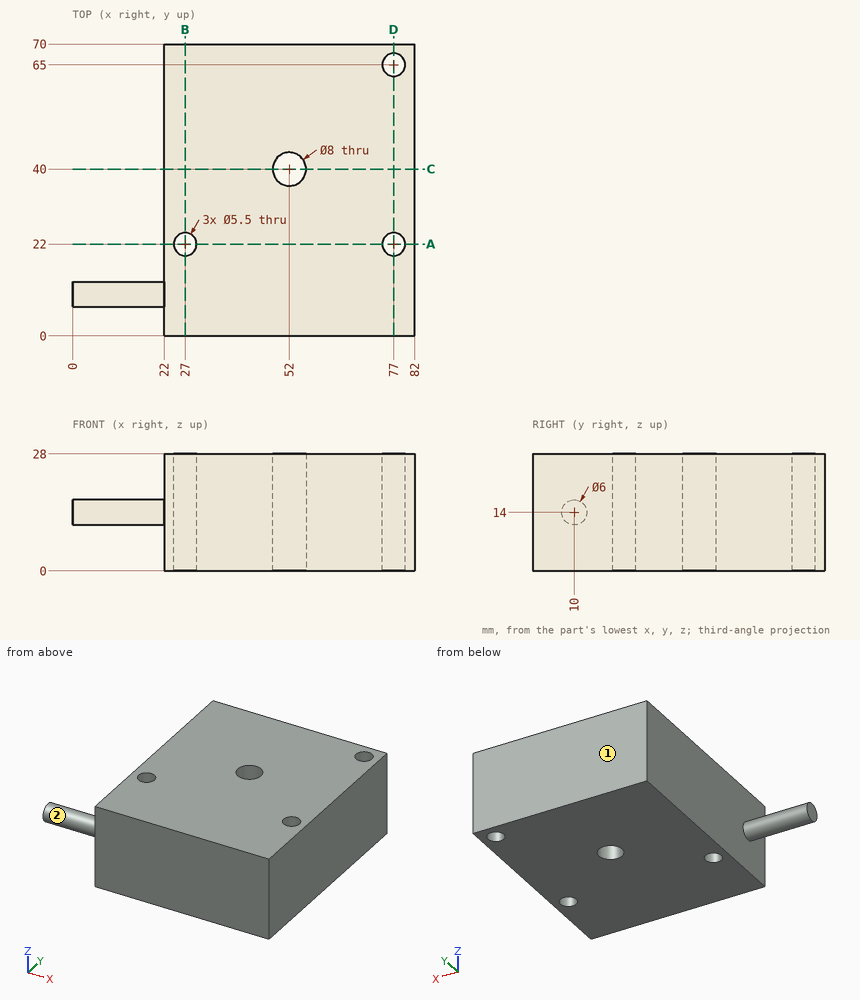
Part print with two shaded views. Sizes in mm from the minimum x, y, z corner. A direction names the side the tool comes from. Round coordinates to 2 decimals unless told otherwise and drop trailing zeros. Write each loop counter-clockwise with the first axis right and the second up, starting at its lowest first coordinate (ties: lowest second). Pieces come first, ordered by that corner, then holes. Notation, with made-up numbers: (-1.75, -9.5) - (4.25, -9.5) arc R21 ccw to (4.25, 28.5) - close; hole circle Ø2 at (50.5, 50.5). An arc over 180 degrees is marked (long way). Answer as CSV lines item,"result".
Q1. Cut at B-B (x = 27). Write the cut outline in (y, z).
Report:
outline,"(0, 0) - (19.25, 0) - (19.25, 28) - (0, 28) - close; (24.75, 0) - (70, 0) - (70, 28) - (24.75, 28) - close"
Q2. Cut at A-A (y = 22). Write the cut outline in (x, z), and give its area (3 significant figures).
Report:
outline,"(22, 0) - (24.25, 0) - (24.25, 28) - (22, 28) - close; (29.75, 0) - (74.25, 0) - (74.25, 28) - (29.75, 28) - close; (79.75, 0) - (82, 0) - (82, 28) - (79.75, 28) - close"
area,"1,370 mm^2"
Q3. Cut at D-D (x = 77). Write the cut outline in (y, z), and give its area (3 significant figures).
Report:
outline,"(0, 0) - (19.25, 0) - (19.25, 28) - (0, 28) - close; (24.75, 0) - (62.25, 0) - (62.25, 28) - (24.75, 28) - close; (67.75, 0) - (70, 0) - (70, 28) - (67.75, 28) - close"
area,"1,650 mm^2"
Q4. Tool access for the marked faces 1 and 2: list every direction of +Z, -Z, +X, -X, +Y, -Y with a clear straight run to the whole face (end or side of a thin tool).
Report:
face 1,"+Z, -Z, +X, -X, +Y"
face 2,"-X"
Q5. Cut at C-C (y = 40). Write the cut outline in (x, z), and give its area (3 significant figures).
Report:
outline,"(22, 0) - (48, 0) - (48, 28) - (22, 28) - close; (56, 0) - (82, 0) - (82, 28) - (56, 28) - close"
area,"1,460 mm^2"
Q6. Drop flat-ended pins along their axis: pin 1 (2 mm diameter, centred on x = 53.5, y = 41.5, fed in from +Z); pin 2 (6 mm diameter, centred on y = 23, z = 14.5, fed in from -X). Give the stop position or say it passes through.
Report:
pin 1,"passes through"
pin 2,"stops at x = 22"
Q7. Drill centre lines: probe 1 along Y at (x, z) = (77, 18.75); probe 2 along Y at (x, z) = (27, 6.75); probe 3 along X at (y, z) = (49, 16.25). Where is each one in solid material? Low to high. Write a range as [from, to].
Report:
probe 1,"y = [0, 19.25], [24.75, 62.25], [67.75, 70]"
probe 2,"y = [0, 19.25], [24.75, 70]"
probe 3,"x = [22, 82]"
